from build123d import *

# Parameters (mm, degrees)
F0_R     = 1.6
F0_W     = 6.4
F0_H     = 3.4
F0_W_2   = 2
F0_H_2   = 6
F1_DEPTH = 3


# Not quite as in the source:
# - ends of sketch curves that miss each other by under 0.0002 mm in the source are joined


with BuildPart() as f1:
    # F0 (on Top) → F1 (new body)
    with BuildSketch(Plane.XY):
        with BuildLine():
            Line((-31.5, 1.5), (-31.5, -1.5))
            Line((-31.5, -1.5), (-28.4, -1.5))
            Line((-28.4, -1.5), (-28.4, -4.7))
            Line((-28.4, -4.7), (-31.5, -4.7))
            Line((-31.5, -4.7), (-31.5, -29.5))
            ThreePointArc((-31.5, -29.5), (-30.6213203436, -31.6213203436), (-28.5, -32.5))
            Line((-28.5, -32.5), (21.468901, -32.5))
            ThreePointArc((21.468901, -32.5), (23.1507874279, -31.9842016914), (24.2543310727, -30.6141720291))
            Line((24.2543310727, -30.6141720291), (31.5, -12.5))
            Line((31.5, -12.5), (31.5, -3.6))
            ThreePointArc((31.5, -3.6), (31.2071067812, -2.8928932188), (30.5, -2.6))
            Line((30.5, -2.6), (17.5, -2.6))
            ThreePointArc((17.5, -2.6), (14.9, 0), (17.5, 2.6))
            Line((17.5, 2.6), (30.5, 2.6))
            ThreePointArc((30.5, 2.6), (31.2071067812, 2.8928932188), (31.5, 3.6))
            Line((31.5, 3.6), (31.5, 12.5))
            Line((31.5, 12.5), (24.2543, 30.6142))
            ThreePointArc((24.2543, 30.6142), (23.1507874279, 31.9842016914), (21.468901, 32.5))
            Line((21.468901, 32.5), (-28.5, 32.5))
            ThreePointArc((-28.5, 32.5), (-30.6213203436, 31.6213203436), (-31.5, 29.5))
            Line((-31.5, 29.5), (-31.5, 4.7))
            Line((-31.5, 4.7), (-28.4, 4.7))
            Line((-28.4, 4.7), (-28.4, 1.5))
            Line((-28.4, 1.5), (-31.5, 1.5))
        make_face()
        with Locations((-28.5, -28.5)):
            Circle(F0_R, mode=Mode.SUBTRACT)
        with Locations((-21.5, -28)):
            Rectangle(F0_W, F0_H, mode=Mode.SUBTRACT)
        with Locations((-21.5, -17)):
            Rectangle(F0_W, F0_H, mode=Mode.SUBTRACT)
        with Locations((-12.5, -25.5)):
            Rectangle(F0_W_2, F0_H_2, mode=Mode.SUBTRACT)
        with Locations((-14.5, -16.8)):
            Circle(F0_R, mode=Mode.SUBTRACT)
        with BuildLine():
            ThreePointArc((-8.0669872236, -29.8000098709), (-8.8535526014, -29.9035641797), (-8.7500018039, -29.1169983396))
            ThreePointArc((-8.7500018039, -29.1169983396), (-8.5669873354, -28.9339800645), (-8.5, -28.68398))
            Line((-8.5, -28.68398), (-8.5, -6.316))
            ThreePointArc((-8.5, -6.316), (-8.5669873354, -6.0659999355), (-8.7500001291, -5.8829872236))
            ThreePointArc((-8.7500001291, -5.8829872236), (-8.8535533906, -5.0964466094), (-8.0669872236, -5.2000001291))
            ThreePointArc((-8.0669872236, -5.2000001291), (-7.8840000645, -5.3830126646), (-7.634, -5.45))
            Line((-7.634, -5.45), (-0.366, -5.45))
            ThreePointArc((-0.366, -5.45), (-0.1159999355, -5.3830126646), (0.0670127764, -5.1999998709))
            ThreePointArc((0.0670127764, -5.1999998709), (0.8535541797, -5.0964473986), (0.7499998709, -5.8830127764))
            ThreePointArc((0.7499998709, -5.8830127764), (0.5669873354, -6.0659999355), (0.5, -6.316))
            Line((0.5, -6.316), (0.5, -28.68397))
            ThreePointArc((0.5, -28.68397), (0.5669873354, -28.9339700645), (0.7500001291, -29.1169827764))
            ThreePointArc((0.7500001291, -29.1169827764), (0.8535533906, -29.9035533906), (0.0669872236, -29.7999998709))
            ThreePointArc((0.0669872236, -29.7999998709), (-0.1159999355, -29.6169873354), (-0.366, -29.55))
            Line((-0.366, -29.55), (-7.634, -29.55001))
            ThreePointArc((-7.634, -29.55001), (-7.8840000645, -29.6169973354), (-8.0669872236, -29.8000098709))
        make_face(mode=Mode.SUBTRACT)
        with Locations((-12.5, -9.5)):
            Rectangle(F0_W_2, F0_H_2, mode=Mode.SUBTRACT)
        with Locations((4.5, -25.5)):
            Rectangle(F0_W_2, F0_H_2, mode=Mode.SUBTRACT)
        with Locations((13.5, -28)):
            Rectangle(F0_W, F0_H, mode=Mode.SUBTRACT)
        with Locations((6.5, -16.8)):
            Circle(F0_R, mode=Mode.SUBTRACT)
        with Locations((13.5, -17)):
            Rectangle(F0_W, F0_H, mode=Mode.SUBTRACT)
        with Locations((20.5, -28.5)):
            Circle(F0_R, mode=Mode.SUBTRACT)
        with Locations((4.5, -9.5)):
            Rectangle(F0_W_2, F0_H_2, mode=Mode.SUBTRACT)
        with Locations((-10.5, 0)):
            Rectangle(F0_W, F0_H, mode=Mode.SUBTRACT)
        with Locations((-12.5, 9.5)):
            Rectangle(F0_W_2, F0_H_2, mode=Mode.SUBTRACT)
        with Locations((-21.5, 17)):
            Rectangle(F0_W, F0_H, mode=Mode.SUBTRACT)
        with Locations((-28.5, 28.5)):
            Circle(F0_R, mode=Mode.SUBTRACT)
        with Locations((-21.5, 28)):
            Rectangle(F0_W, F0_H, mode=Mode.SUBTRACT)
        with Locations((-14.5, 16.8)):
            Circle(F0_R, mode=Mode.SUBTRACT)
        with BuildLine():
            ThreePointArc((-8.0669772236, 5.1999911291), (-8.8535424247, 5.0964366435), (-8.7499922369, 5.8830024104))
            ThreePointArc((-8.7499922369, 5.8830024104), (-8.5669772104, 6.066020152), (-8.49999, 6.31602))
            Line((-8.49999, 6.31602), (-8.49999, 28.684))
            ThreePointArc((-8.49999, 28.684), (-8.5669773354, 28.9340000645), (-8.7499901291, 29.1170127764))
            ThreePointArc((-8.7499901291, 29.1170127764), (-8.8535432138, 29.9035535674), (-8.0669772236, 29.7999998709))
            ThreePointArc((-8.0669772236, 29.7999998709), (-7.8839900645, 29.6169873354), (-7.63399, 29.55))
            Line((-7.63399, 29.55), (-0.36599, 29.55))
            ThreePointArc((-0.36599, 29.55), (-0.1159899355, 29.6169873354), (0.0670227764, 29.8000001291))
            ThreePointArc((0.0670227764, 29.8000001291), (0.853564003, 29.9035527782), (0.7500103039, 29.1169874736))
            ThreePointArc((0.7500103039, 29.1169874736), (0.5669973354, 28.9340000645), (0.50001, 28.684))
            Line((0.50001, 28.684), (0.50001, 6.316031))
            ThreePointArc((0.50001, 6.316031), (0.5669973354, 6.0660309355), (0.7500101291, 5.8830182236))
            ThreePointArc((0.7500101291, 5.8830182236), (0.8535633906, 5.0964466094), (0.0669972236, 5.2000001291))
            ThreePointArc((0.0669972236, 5.2000001291), (-0.1159899355, 5.3830126646), (-0.36599, 5.45))
            Line((-0.36599, 5.45), (-7.63399, 5.449991))
            ThreePointArc((-7.63399, 5.449991), (-7.8839900645, 5.3830036646), (-8.0669772236, 5.1999911291))
        make_face(mode=Mode.SUBTRACT)
        with Locations((-12.5, 25.5)):
            Rectangle(F0_W_2, F0_H_2, mode=Mode.SUBTRACT)
        with Locations((4.5, 9.5)):
            Rectangle(F0_W_2, F0_H_2, mode=Mode.SUBTRACT)
        with Locations((6.5, 16.8)):
            Circle(F0_R, mode=Mode.SUBTRACT)
        with Locations((13.5, 17)):
            Rectangle(F0_W, F0_H, mode=Mode.SUBTRACT)
        with Locations((4.5, 25.5)):
            Rectangle(F0_W_2, F0_H_2, mode=Mode.SUBTRACT)
        with Locations((13.5, 28)):
            Rectangle(F0_W, F0_H, mode=Mode.SUBTRACT)
        with Locations((20.5, 28.5)):
            Circle(F0_R, mode=Mode.SUBTRACT)
    extrude(amount=F1_DEPTH)


solid = f1.part
Can you work these out from the model? Positions are in its coordinate system, mm. A direction names the side the tool comes from. Give positions to 0.01 mm unless a question says otherwise; leave off trailing zeros. Loops run counter-clockwise (first coordinate to the right, second up) from the corner with the lowest first, then second, coordinate; pieces in that order, holes last. Notation, with made-up numbers: (89.5, 26) - (136.5, 26) arc R23 ccw to (136.5, 37) - close; hole circle Ø2 at (46, 9). An arc over 180 degrees is marked (long way). Return JSON: item names as keys, results as strings.
1. For faces 1 (the face through (0, 0, 3)), 2 (the face through (-11.5, -10, 1)), 3 (the face through (-28.4, -3, 1)), which set-ups out of +Z, -Z, +X, -X, +Y, -Y let a thin tool reach every point of the face, with its end or its side?
Output values:
{"face 1": "+Z, +X, -X, +Y, -Y", "face 2": "+Z, -Z", "face 3": "+Z, -Z, -X"}
2. I want a section at B-B on x = -10. Please give me the cut outline in (y, z).
Output values:
{"outline": "(-32.5, 0) - (-1.7, 0) - (-1.7, 3) - (-32.5, 3) - close; (1.7, 0) - (32.5, 0) - (32.5, 3) - (1.7, 3) - close"}
3. I want a section at C-C on y = 10. Please give me the cut outline in (x, z).
Output values:
{"outline": "(-31.5, 0) - (-13.5, 0) - (-13.5, 3) - (-31.5, 3) - close; (-11.5, 0) - (-8.5, 0) - (-8.5, 3) - (-11.5, 3) - close; (0.5, 0) - (3.5, 0) - (3.5, 3) - (0.5, 3) - close; (5.5, 0) - (31.5, 0) - (31.5, 3) - (5.5, 3) - close"}
4. I want a section at D-D on x = 6.5. Please give me the cut outline in (y, z), and give its area (3 significant figures).
Output values:
{"outline": "(-32.5, 0) - (-18.4, 0) - (-18.4, 3) - (-32.5, 3) - close; (-15.2, 0) - (15.2, 0) - (15.2, 3) - (-15.2, 3) - close; (18.4, 0) - (32.5, 0) - (32.5, 3) - (18.4, 3) - close", "area": "176 mm²"}
5. I'm going to push flat-ended pins straight in: pin 1 Ø3 at (x, y) = (-14.5, -16.8) entering from -Z; pin 2 Ø1.5 at (y, z) = (17.5, 2) entering from +X. Where does each tip first touch, or does it pass through?
Output values:
{"pin 1": "passes through", "pin 2": "stops at x = 29.8"}
6. If I drill on line 1 (X direction, y = -8.5, z = 2); line 2 (Y direction, x = 6.5, z = 2.2); line 3 (Y direction, x = -7, z = 0.3), over which ranges is the centre line in solid material (lowest first)?
Output values:
{"line 1": "x = -31.5 to -13.5, -11.5 to -8.5, 0.5 to 3.5, 5.5 to 31.5", "line 2": "y = -32.5 to -18.4, -15.2 to 15.2, 18.4 to 32.5", "line 3": "y = -32.5 to -29.55, -5.45 to 5.45, 29.55 to 32.5"}
7. I want a section at A-A on y = 16.8. Please give me the cut outline in (x, z).
Output values:
{"outline": "(-31.5, 0) - (-24.7, 0) - (-24.7, 3) - (-31.5, 3) - close; (-18.3, 0) - (-16.1, 0) - (-16.1, 3) - (-18.3, 3) - close; (-12.9, 0) - (-8.5, 0) - (-8.5, 3) - (-12.9, 3) - close; (0.5, 0) - (4.9, 0) - (4.9, 3) - (0.5, 3) - close; (8.1, 0) - (10.3, 0) - (10.3, 3) - (8.1, 3) - close; (16.7, 0) - (29.78, 0) - (29.78, 3) - (16.7, 3) - close"}
8. We'd pull the mould along X, two halves only. Please class faces 4 (the face through (3.5, -26, 1)), 5 (the face through (3.5, 25, 1)), 6 (the face through (-30, -4.7, 1)), 7 (the face through (-31.5, -17, 1)): +X half, -X half, draft (parallel to the pull), parting line (faces both ways), or undercut.
Output values:
{"face 4": "undercut", "face 5": "undercut", "face 6": "draft", "face 7": "-X half"}
